```python
from build123d import *

# Parameters (mm, degrees)
BODY_DEPTH                                      = 32
BODY_DEPTH_BACK                                 = 15
PIVOT_HOLE_DEPTH                                = 40.272286666
PIVOT_HOLE_DEPTH_BACK                           = 40.272286666
PIVOT_HOLE_SKETCH_R                             = 4.05
OUTSIDE_SHAPE_CUT_OUT_DEPTH                     = 40.272286666
OUTSIDE_SHAPE_CUT_OUT_DEPTH_BACK                = 40.272286666
OUTSIDE_SHAPE_CUT_OUT_SKETCH_W                  = 49
OUTSIDE_SHAPE_CUT_OUT_SKETCH_H                  = 22
INSIDE_START                                    = 17.25
INSIDE_SHAPE_CUT_OUT_DEPTH                      = 34.5
F_2_START                                       = -11.75
F_2_LATERAL_SLOTS_ORIENTED_LONGITUDINALLY_DEPTH = 3.5


with BuildPart() as part:
    # Profile Sketch → Body (new, two sides: drawn at the far end of the back side and taken through both)
    with BuildSketch(Plane.XY.offset(-BODY_DEPTH_BACK)):
        Polygon((-19.5, -11.75), (19.5, -11.75), (19.5, 8.25), (17.25, 8.25), (17.25, -8.25), (-17.25, -8.25), (-17.25, 8.25), (-19.5, 8.25), align=None)
    extrude(amount=BODY_DEPTH + BODY_DEPTH_BACK)

    # Pivot Hole Sketch → Pivot Hole (cut, two sides: drawn at the far end of the back side and taken through both)
    with BuildSketch(Plane(origin=(0, 0, 0), x_dir=(0, 0, -1), z_dir=(1, 0, 0)).offset(-PIVOT_HOLE_DEPTH_BACK)):
        with Locations((0, -1.75)):
            Circle(PIVOT_HOLE_SKETCH_R)
    extrude(amount=PIVOT_HOLE_DEPTH + PIVOT_HOLE_DEPTH_BACK, mode=Mode.SUBTRACT)

    # Outside Shape Cut Out Sketch → Outside Shape Cut Out (cut, two sides: drawn at the far end of the back side and taken through both)
    with BuildSketch(Plane(origin=(0, 0, 0), x_dir=(0, 0, -1), z_dir=(1, 0, 0)).offset(-OUTSIDE_SHAPE_CUT_OUT_DEPTH_BACK)):
        with Locations((-9.5, -2.75)):
            Rectangle(OUTSIDE_SHAPE_CUT_OUT_SKETCH_W, OUTSIDE_SHAPE_CUT_OUT_SKETCH_H)
        with BuildLine():
            Line((-27.649101987, 3.819656009), (-5.267826876, 6.75))
            ThreePointArc((-5.267826876, 6.75), (-3.57284062, 7.589957703), (-1.75, 8.095684334))
            Line((-1.75, 8.095684334), (-1.25, 6.15))
            Line((-1.25, 6.15), (1.25, 6.15))
            Line((1.25, 6.15), (1.75, 8.095684334))
            ThreePointArc((1.75, 8.095684334), (7.071067812, 5.321067812), (9.845684334, 0))
            Line((9.845684334, 0), (7.9, -0.5))
            Line((7.9, -0.5), (7.9, -3))
            Line((7.9, -3), (9.845684334, -3.5))
            ThreePointArc((9.845684334, -3.5), (6.422616289, -9.414854858), (0, -11.75))
            Line((0, -11.75), (-32, -11.75))
            Line((-32, -11.75), (-32, -1.138031619))
            ThreePointArc((-32, -1.138031619), (-30.758025408, 2.160035244), (-27.649101987, 3.819656009))
        make_face(mode=Mode.SUBTRACT)
    extrude(amount=OUTSIDE_SHAPE_CUT_OUT_DEPTH + OUTSIDE_SHAPE_CUT_OUT_DEPTH_BACK, mode=Mode.SUBTRACT)

    # Inside Shape Cut Out Sketch → Inside Shape Cut Out (cut)
    with BuildSketch(Plane(origin=(0, 0, 0), x_dir=(0, 0, -1), z_dir=(1, 0, 0)).offset(INSIDE_START)):
        Polygon((-29, -9.75), (-29, -11.75), (-32, -11.75), (-32, -10.75), (-30.5, -10.75), (-30.5, -9.75), align=None)
        Polygon((-9.5, -8.25), (-5, -10.75), (-5, -11.75), (7.599342077, -11.75), (7.599342077, -8.25), align=None)
    extrude(amount=-INSIDE_SHAPE_CUT_OUT_DEPTH, mode=Mode.SUBTRACT)

    # 2 Lateral Slots Oriented Longitudinally: read off the stored shape, not the designer's step
    # 2 Lateral Slots Oriented Longitudina 2 → 2 Lateral Slots Oriented Longitudinally (cut)
    with BuildSketch(Plane(origin=(0, 0, 0), x_dir=(1, 0, 0), z_dir=(0, 1, 0)).offset(F_2_START)):
        with BuildLine():
            Line((10.15, -25.35), (10.15, -22.65))
            ThreePointArc((10.15, -22.65), (8, -20.5), (5.85, -22.65))
            Line((5.85, -22.65), (5.85, -25.35))
            ThreePointArc((5.85, -25.35), (8, -27.5), (10.15, -25.35))
        make_face()
        with BuildLine():
            Line((-5.85, -25.35), (-5.85, -22.65))
            ThreePointArc((-5.85, -22.65), (-8, -20.5), (-10.15, -22.65))
            Line((-10.15, -22.65), (-10.15, -25.35))
            ThreePointArc((-10.15, -25.35), (-8, -27.5), (-5.85, -25.35))
        make_face()
    extrude(amount=F_2_LATERAL_SLOTS_ORIENTED_LONGITUDINALLY_DEPTH, mode=Mode.SUBTRACT)

    # 2 Lateral Slots Oriented Longitudina 3: loft between two sections, ruled curve by curve
    f_2_lateral_slots_oriented_longitudina_3_from = [
        Edge.make_three_point_arc((10.15, -10.8, 22.65), (9.52027958, -10.8, 21.12972042), (8, -10.8, 20.5)),
        Edge.make_three_point_arc((8, -10.8, 20.5), (6.47972042, -10.8, 21.12972042), (5.85, -10.8, 22.65)),
        Edge.make_three_point_arc((5.85, -10.8, 25.35), (6.47972042, -10.8, 26.87027958), (8, -10.8, 27.5)),
        Edge.make_three_point_arc((8, -10.8, 27.5), (9.52027958, -10.8, 26.87027958), (10.15, -10.8, 25.35)),
        Edge.make_line((5.85, -10.8, 22.65), (5.85, -10.8, 25.35)),
        Edge.make_line((10.15, -10.8, 22.65), (10.15, -10.8, 25.35)),
    ]
    f_2_lateral_slots_oriented_longitudina_3_to = [
        Edge.make_three_point_arc((12.7, -8.25, 22.65), (11.323401872, -8.25, 19.326598128), (8, -8.25, 17.95)),
        Edge.make_three_point_arc((8, -8.25, 17.95), (4.676598128, -8.25, 19.326598128), (3.3, -8.25, 22.65)),
        Edge.make_three_point_arc((3.3, -8.25, 25.35), (4.676598128, -8.25, 28.673401872), (8, -8.25, 30.05)),
        Edge.make_three_point_arc((8, -8.25, 30.05), (11.323401872, -8.25, 28.673401872), (12.7, -8.25, 25.35)),
        Edge.make_line((3.3, -8.25, 22.65), (3.3, -8.25, 25.35)),
        Edge.make_line((12.7, -8.25, 22.65), (12.7, -8.25, 25.35)),
    ]
    f_2_lateral_slots_oriented_longitudina_3 = Solid(Shell([*[Face.make_surface_from_curves(f_2_lateral_slots_oriented_longitudina_3_from[k], f_2_lateral_slots_oriented_longitudina_3_to[k]) for k in range(6)], Face(Wire(f_2_lateral_slots_oriented_longitudina_3_from)), Face(Wire(f_2_lateral_slots_oriented_longitudina_3_to))]))
    add(f_2_lateral_slots_oriented_longitudina_3, mode=Mode.SUBTRACT)

    # 2 Lateral Slots Oriented Longitudina 4: loft between two sections, ruled curve by curve
    f_2_lateral_slots_oriented_longitudina_4_from = [
        Edge.make_three_point_arc((-5.85, -10.8, 22.65), (-6.47972042, -10.8, 21.12972042), (-8, -10.8, 20.5)),
        Edge.make_three_point_arc((-8, -10.8, 20.5), (-9.52027958, -10.8, 21.12972042), (-10.15, -10.8, 22.65)),
        Edge.make_three_point_arc((-10.15, -10.8, 25.35), (-9.52027958, -10.8, 26.87027958), (-8, -10.8, 27.5)),
        Edge.make_three_point_arc((-8, -10.8, 27.5), (-6.47972042, -10.8, 26.87027958), (-5.85, -10.8, 25.35)),
        Edge.make_line((-10.15, -10.8, 22.65), (-10.15, -10.8, 25.35)),
        Edge.make_line((-5.85, -10.8, 22.65), (-5.85, -10.8, 25.35)),
    ]
    f_2_lateral_slots_oriented_longitudina_4_to = [
        Edge.make_three_point_arc((-3.3, -8.25, 22.65), (-4.676598128, -8.25, 19.326598128), (-8, -8.25, 17.95)),
        Edge.make_three_point_arc((-8, -8.25, 17.95), (-11.323401872, -8.25, 19.326598128), (-12.7, -8.25, 22.65)),
        Edge.make_three_point_arc((-12.7, -8.25, 25.35), (-11.323401872, -8.25, 28.673401872), (-8, -8.25, 30.05)),
        Edge.make_three_point_arc((-8, -8.25, 30.05), (-4.676598128, -8.25, 28.673401872), (-3.3, -8.25, 25.35)),
        Edge.make_line((-12.7, -8.25, 22.65), (-12.7, -8.25, 25.35)),
        Edge.make_line((-3.3, -8.25, 22.65), (-3.3, -8.25, 25.35)),
    ]
    f_2_lateral_slots_oriented_longitudina_4 = Solid(Shell([*[Face.make_surface_from_curves(f_2_lateral_slots_oriented_longitudina_4_from[k], f_2_lateral_slots_oriented_longitudina_4_to[k]) for k in range(6)], Face(Wire(f_2_lateral_slots_oriented_longitudina_4_from)), Face(Wire(f_2_lateral_slots_oriented_longitudina_4_to))]))
    add(f_2_lateral_slots_oriented_longitudina_4, mode=Mode.SUBTRACT)


solid = part.part
```
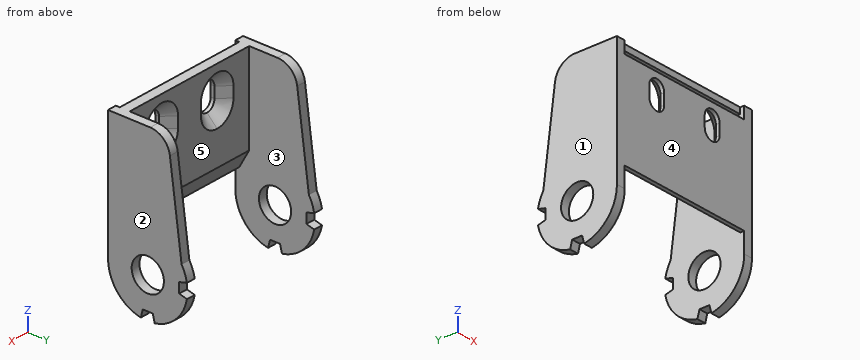
Check sheet for the modelled part. Datum: model origin and axes. Units: mm. Face numbers are marked on the shaded views. A direction names the side the tool comes from. Give positions to 0.01 mm unless a question says otherwise; leave off trailing zeros. Order: outer loops, then holes, each group sorted by start corner. A loop starts at its lowest first (then second) coordinate and runs counter-clockwise, first axis right, second up. Notation, with made-up numbers: M 38,69 L 59,69 A14 cw 59,91 Z; hole C 15,76 d9. An arc over 180 degrees is marked long. Answer in a Markdown table with one row per item. Add a question column.
Q1. Sectioned sample at A-A, the plane y = -1.75. Record the boundary of the cut face in (x, z), and give its area (3 significant figures).
Q2. Access from +Z, -Z, +X, -X, +Y, -Y to the whole of each face (thin tool, end or side, straight path). Record for the marked faces 4 and 5.
Q3. Thickness scan on L1, parallel to Z at x = 18, y = -1.75; L2, parallel to X at y = -7.25, z = 0.5; L3, parallel to X at y = -8.5, z = 22.5. Record the ranges inside material, lowest first.
Q4. Sectioned sample at C-C, the plane z = -3. Record the boundary of the cut face in (x, y), and give its area (3 significant figures).
Q5. Gauge pin test, flat ends, axial feed: pin 1 Ø1.1 at (x, y) = (6, -10) entering from -Z; pin 2 Ø1.8 at (x, z) = (-18.5, 0) entering from +Y; pin 3 Ø0.8 at (x, z) = (0.5, 30) entering from -Y. Record the tip position at first contact, or that the pin passes through.
Q6. Sectioned sample at D-D, the plane z = 10. Record the boundary of the cut face in (x, y), and give its area (3 significant figures).
Q7. Release check for a two-part mould opening along X. For the marked faces 1, 2 and 3 record: released by +X, released by -X, zero draft, split by the parting line, or undercut.
Q8. Sectioned sample at B-B, the plane x = 16. Record the boundary of the cut face in (y, z), and give its area (3 significant figures).
Verdict:
| question | item | result |
|---|---|---|
| 1 | outline | M -19.5,-7.9 L -17.25,-7.9 L -17.25,-4.05 L -19.5,-4.05 Z; M -19.5,4.05 L -17.25,4.05 L -17.25,32 L -19.5,32 Z; M 17.25,-7.9 L 19.5,-7.9 L 19.5,-4.05 L 17.25,-4.05 Z; M 17.25,4.05 L 19.5,4.05 L 19.5,32 L 17.25,32 Z |
| 1 | area | 143 mm² |
| 2 | face 4 | +Z, -Z, +X, -X, -Y |
| 2 | face 5 | +Z, -Z, +Y |
| 3 | L1 | -7.9 to -4.05, 4.05 to 32 |
| 3 | L2 | -19.5 to -17.25, 17.25 to 19.5 |
| 3 | L3 | -19.5 to -12.45, -3.55 to 3.55, 12.45 to 19.5 |
| 4 | outline | M -19.5,-11.29 L -17.25,-11.29 L -17.25,-4.47 L -19.5,-4.47 Z; M -19.5,0.97 L -17.25,0.97 L -17.25,7.79 L -19.5,7.79 Z; M 17.25,-11.29 L 19.5,-11.29 L 19.5,-4.47 L 17.25,-4.47 Z; M 17.25,0.97 L 19.5,0.97 L 19.5,7.79 L 17.25,7.79 Z |
| 4 | area | 61.4 mm² |
| 5 | pin 1 | z = 5.36 |
| 5 | pin 2 | y = 6.15 |
| 5 | pin 3 | y = -9.75 |
| 6 | outline | M -19.5,-11.75 L 19.5,-11.75 L 19.5,6.13 L 17.25,6.13 L 17.25,-8.25 L -17.25,-8.25 L -17.25,6.13 L -19.5,6.13 Z |
| 6 | area | 201 mm² |
| 7 | face 1 | released by -X |
| 7 | face 2 | released by +X |
| 7 | face 3 | undercut |
| 8 | outline | M -11.75,5 L -10.75,5 L -8.25,9.5 L -8.25,32 L -10.75,32 L -10.75,30.5 L -9.75,30.5 L -9.75,29 L -11.75,29 Z |
| 8 | area | 84.4 mm² |
